Source: CAD feature listing. Evaluate the final solid. Frame: model axes, mm. Face numbers are marked on the shaded views. Give positions to 0.01 mm unless a question says otherwise; leave off trailing zeros. Loops run counter-clockwise (first coordinate to the right, second up) from the corner with the lowest first, then second, coordinate; pieces in that order, holes last. Notation, with made-up numbers: (66, 28.5) -> (111, 28.5) arc R25 ccw to (111, 51.5) -> close; hole circle Ø6 at (33.25, 88). An arc over 180 degrees is marked (long way). Return JSON: item names as keys, results as strings. Group by question number.
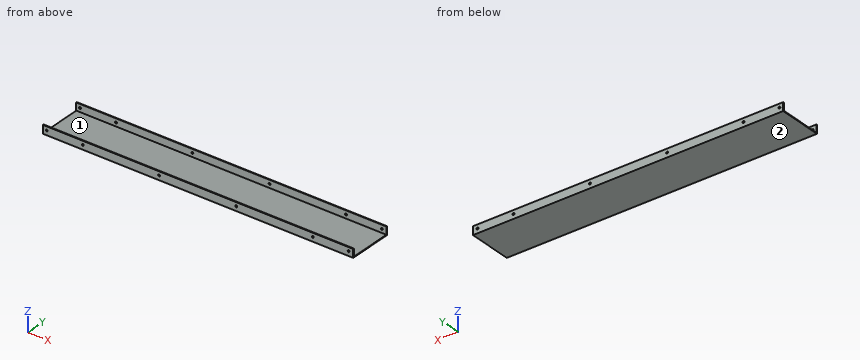
```python
from build123d import *

# Parameters (mm, degrees)
SKETCH_1_W          = 820
SKETCH_1_H          = 116
EXTRUDE_1_DEPTH     = 2
SKETCH_2_W          = 820
SKETCH_2_H          = 2
EXTRUDE_2_DEPTH     = 20
SKETCH_3_R          = 2.5
CUT_EXTRUDE_2_DEPTH = 116


with BuildPart() as part:
    # 草图1 → 凸台-拉伸1 (new body)
    with BuildSketch(Plane.XY):
        with Locations((395.921840051, 50.211278088)):
            Rectangle(SKETCH_1_W, SKETCH_1_H)
    extrude(amount=EXTRUDE_1_DEPTH)

    # 草图2 → 凸台-拉伸2 (add)
    with BuildSketch(Plane.XY.offset(2)):
        with Locations((395.921840051, 107.211278088)):
            Rectangle(SKETCH_2_W, SKETCH_2_H)
        with Locations((395.921840051, -6.788721912)):
            Rectangle(SKETCH_2_W, SKETCH_2_H)
    extrude(amount=EXTRUDE_2_DEPTH)

    # 草图3 → 切除-拉伸2 (cut)
    with BuildSketch(Plane(origin=(0, 108.211278088, 0), x_dir=(1, 0, 0), z_dir=(0, 1, 0))):
        with Locations(Location((698.921840051, -12, 0), (0, 0, 270))):
            Circle(SKETCH_3_R)
        with Locations(Location((793.921840051, -12, 0), (0, 0, 270))):
            Circle(SKETCH_3_R)
        with Locations(Location((-4.078159949, -12, 0), (0, 0, 270))):
            Circle(SKETCH_3_R)
        with Locations(Location((90.921840051, -12, 0), (0, 0, 270))):
            Circle(SKETCH_3_R)
        with Locations(Location((292.921840051, -12, 0), (0, 0, 270))):
            Circle(SKETCH_3_R)
        with Locations(Location((496.921840051, -12, 0), (0, 0, 270))):
            Circle(SKETCH_3_R)
    extrude(amount=-CUT_EXTRUDE_2_DEPTH, mode=Mode.SUBTRACT)


solid = part.part
```
1) Contact query for a flat-ended pin moving along its axis: P1, Ø5, axis at x = 461.5, y = 29, coming from the +Z side. Output: stop coordinate, or through.
2) Cut plane B-B on x = 410. Return loops of the section in (y, z), then the cut area to 3 significant figures.
3) Material intervals for line 1 (Y direction, x = 745.5, z = 10.5); line 2 (Z direction, x = 733, y = 67), sorted ascending.
4) Cut plane C-C on y = 40. Return loops of the section in (x, z).
5) Mould query, pull axis Y, two halves, no side actions, for the marked faces 1 and 2. Classes: released by +Y, released by -Y, zero draft, split by the parting line, or undercut.
6) Cut plane A-A on z = 18.25. Return loops of the section in (x, y), then the cut area to 3 significant figures.
Calculated:
{
 "1": {"P1": "z = 2"},
 "2": {"outline": "(-7.79, 0) -> (108.21, 0) -> (108.21, 22) -> (106.21, 22) -> (106.21, 2) -> (-5.79, 2) -> (-5.79, 22) -> (-7.79, 22) -> close", "area": "312 mm2"},
 "3": {"line 1": "-7.79 to -5.79, 106.21 to 108.21", "line 2": "0 to 2"},
 "4": {"outline": "(-14.08, 0) -> (805.92, 0) -> (805.92, 2) -> (-14.08, 2) -> close"},
 "5": {"face 1": "undercut", "face 2": "zero draft"},
 "6": {"outline": "(-14.08, -7.79) -> (805.92, -7.79) -> (805.92, -5.79) -> (-14.08, -5.79) -> close; (-14.08, 106.21) -> (805.92, 106.21) -> (805.92, 108.21) -> (-14.08, 108.21) -> close", "area": "3,280 mm2"}
}
